Part model, mm, in its own coordinate system. Coordinates: 2 decimals unless noted, no trailing zeros. Loops run counter-clockwise (first coordinate to the right, second up) from the corner with the lowest first, then second, coordinate; pieces in that order, holes last. Notation, with made-up numbers: (-21.75, 53) -> (15.25, 53) arc R22 ccw to (15.25, 71) -> close; hole circle Ø8 at (-2, -8). An arc over 180 degrees is marked (long way). Use one line per item in the form item = value. Start each with the question number.
(1) Mould opens along X. For faces 1 (the cylindrical face through (-1.873, -9.819, 0.409)), 2 (the flat face through (-15, 0, -3.81)), 3 (the flat face through (-14, 0, -29.21)) say: +X half, -X half, draft (parallel to the pull), parting line (faces both ways), or undercut.
(2) Band-saw the part on B-B on z = -11. Give the cut face in (x, y).
(3) Pin check, flat tips, straight feed: P1, Ø6, axis at x = -7, y = -7, coming from the +Z side; P2, Ø5, axis at y = 6, z = 3, coming from the -X side; P3, Ø6, axis at y = -6, z = -4, coming from the -X side; P4, Ø12, axis at x = -18, z = 2.5, coming from the -Y side. Stop position of each tip, or through.
(4) Drill centre lines: L1, parallel to Y at x = -14, z = 21; L2, parallel to Z at x = -20, y = 7; L3, parallel to X at y = -13, z = 20.5. Where is each one in solid material? Low to high. Write a range as [from, to].
(5) Band-saw the part on C-C on z = 24. Give the cut face in (x, y), then the cut area to 3 significant figures.
(6) Band-saw the part on A-A on y = 0. Give the cut face in (x, z), then the cut area to 3 significant figures.
```python
from build123d import *

# Parameters (mm, degrees)
F0_W     = 16.1361260527
F0_H     = 63.5
F2_R     = 14.8058887609
F3_DEPTH = 38.1


# Not quite as in the source:
# - a fillet or chamfer that OpenCascade refuses, or shapes differently, is made with other operations: its cross-section is extruded or revolved along the edge and cut away or added


with BuildPart() as f1:
    # F0 (on Front) → F1 (revolve)
    with BuildSketch(Plane.XZ):
        with Locations((-22.7458069295, 2.539942234)):
            Rectangle(F0_W, F0_H)
    revolve(axis=Axis((-14.6777439032, 0, 2.539942234), (0, 0, -1)))

    # F2 (on face) → F3 (cut)
    with BuildSketch(Plane.XY.offset(34.289942234)):
        with Locations((-14.6777439032, 0)):
            Circle(F2_R)
    extrude(amount=-F3_DEPTH, mode=Mode.SUBTRACT)

    # F4: chamfer of 5.08 on 1 edges, made by hand

    # F4_s1 → F4_t2 (revolve, cut)
    with BuildSketch(Plane.XZ):
        Polygon((-30.8138699559, 29.209942234), (-25.7338699559, 34.289942234), (-30.8138699559, 34.289942234), align=None)
    revolve(axis=Axis((-14.6777439032, 0, 34.289942234), (0, 0, -1)), mode=Mode.SUBTRACT)


solid = f1.part
```
A:
q1.face_1 = parting line
q1.face_2 = undercut
q1.face_3 = draft
q2.outline = circle Ø32.27 at (-14.68, 0)
q3.P1 = -3.81
q3.P2 = -30.43
q3.P3 = -30.53
q3.P4 = -16.14
q4.L1 = [-16.12, -14.79], [14.79, 16.12]
q4.L2 = [-29.21, -3.81]
q4.L3 = [-24.24, -21.76], [-7.59, -5.12]
q5.outline = circle Ø32.27 at (-14.68, 0); hole circle Ø29.61 at (-14.68, 0)
q5.area = 129 mm²
q6.outline = (-30.81, -29.21) -> (1.46, -29.21) -> (1.46, 29.21) -> (0.13, 30.54) -> (0.13, -3.81) -> (-29.48, -3.81) -> (-29.48, 30.54) -> (-30.81, 29.21) -> close
q6.area = 909 mm²
